The model under review builds one solid part; all positions refer to its coordinate system, in mm. Round coordinates to 2 decimals unless told otherwise and drop trailing zeros. Order: outer loops, then holes, each group sorted by start corner. A loop starts at its lowest first (then second) coordinate and runs counter-clockwise, first axis right, second up.
Solid Edge part; units mm, degrees
sketch "Sketch1" plane through (0, 0, 0) normal (0, 0, 1) x (1, 0, 0)
  line L0 (-6.1009, 4.0673) -> (-6.5728, -3.2499)
  line L1 (-6.5728, -3.2499) -> (-0.4719, -7.3171)
  line L2 (-0.4719, -7.3171) -> (6.1009, -4.0673)
  line L3 (6.1009, -4.0673) -> (6.5728, 3.2499)
  line L4 (6.5728, 3.2499) -> (0.4719, 7.3171)
  line L5 (0.4719, 7.3171) -> (-6.1009, 4.0673)
extrude "Protrusion1" add sketch "Sketch1" against normal blind 120
sketch "Sketch2" plane through (0, 0, -2) normal (0, 0, 1) x (-0.8964, -0.4432, 0)
  circle A0 centre (0, 0) radius 5.5
  circle A1 centre (0, 0) radius 13.1424
extrude "ExtrudedCutout_1" cut sketch "Sketch2" against normal blind 2
sketch "Sketch3" plane through (0, 0, -118) normal (0, 0, -1) x (0.8964, 0.4432, 0)
  circle A0 centre (0, 0) radius 5.5
  circle A1 centre (0, 0) radius 13.1424
extrude "ExtrudedCutout_2" cut sketch "Sketch3" against normal blind 2
properties part number "BumbleB0452"
(1) Consider section A-A (z = -81). Write out the cut boundary in (x, y).
Data:
outline: (-6.57, -3.25) - (-0.47, -7.32) - (6.1, -4.07) - (6.57, 3.25) - (0.47, 7.32) - (-6.1, 4.07) - close
(2) Draft analysis for pull direction Z (two halves, no side actions). For faces 1 (the flat face through (-5, -3, -2)), 2 (the flat face through (2.8, -5.7, -119)), 3 (the flat face through (0, 0, 0)), state which applies: pulls with the +Z half, pulls with the -Z half, needs draft (parallel to the pull), parting line crosses it, or undercut.
Data:
face 1: undercut
face 2: needs draft
face 3: pulls with the +Z half
(3) To check wall thickness, follow probe 1 along Z at (x, y) = (6.25, 3.25); probe 2 along X at (y, z) = (-5.5, -66.5); probe 3 along X at (y, z) = (-2.5, -103). State the ranges of each line that lie inside material, in increasing order.
Data:
probe 1: z = -120 to -118, -116 to -4, -2 to 0
probe 2: x = -3.2 to 3.2
probe 3: x = -6.52 to 6.2
(4) Insertion check: pin 1 (1 mm diameter, centred on x = -0.5, z = -53, fed in from +Y); pin 2 (3 mm diameter, centred on x = -2, z = -80.5, fed in from -Y); pin 3 (6 mm diameter, centred on x = 5, z = -74.5, fed in from -Y). Each pin has a flat end and moves straight along its axis. Give the tip position at first contact, or say it passes through.
Data:
pin 1: stops at y = 7.08
pin 2: stops at y = -7.3
pin 3: stops at y = -6.09
(5) Consider section B-B (y = 0). Write out the cut boundary in (x, z).
Data:
outline: (-6.36, -120) - (6.36, -120) - (6.36, -118) - (5.5, -118) - (5.5, -116) - (6.36, -116) - (6.36, -4) - (5.5, -4) - (5.5, -2) - (6.36, -2) - (6.36, 0) - (-6.36, 0) - (-6.36, -2) - (-5.5, -2) - (-5.5, -4) - (-6.36, -4) - (-6.36, -116) - (-5.5, -116) - (-5.5, -118) - (-6.36, -118) - close
